from build123d import *

# Parameters (mm, degrees)
SKETCH1_R           = 75
BOSS_EXTRUDE1_DEPTH = 100
SHELL1_T            = -5
SKETCH3_R           = 20
SKETCH2_R           = 30
FILLET2_R           = 10


# Read off the part's stored shape, not the designer's step: Shell2
with BuildPart() as part:
    # Sketch1 → Boss-Extrude1 (new body)
    with BuildSketch(Plane(origin=(0, 0, 0), x_dir=(1, 0, 0), z_dir=(0, 1, 0))):
        with Locations(Location((0, 0, 0), (0, 0, 270))):
            Circle(SKETCH1_R)
    extrude(amount=BOSS_EXTRUDE1_DEPTH)

    # Shell1
    shell1_openings = [part.faces().sort_by_distance(p)[0] for p in [
        (0, 100, 0),
    ]]
    offset(amount=SHELL1_T, openings=shell1_openings, kind=Kind.INTERSECTION)

    # Sketch3 → Loft1 section 0
    with BuildSketch(Plane(origin=(0, 100, 0), x_dir=(1, 0, 0), z_dir=(0, 1, 0))):
        Circle(SKETCH3_R)
    # Sketch2 → Loft1 section 1
    with BuildSketch(Plane.XZ):
        Circle(SKETCH2_R)
    loft()

    # Shell2 outline → Shell2 (revolve, cut)
    with BuildSketch(Plane.XY):
        Polygon((0, 0), (24.975062189, 0), (14.975062189, 100), (0, 100), align=None)
    revolve(axis=Axis((0, 0, 0), (0, 1, 0)), mode=Mode.SUBTRACT)

    # Fillet1
    # an asymmetric fillet: 30, 5 mm, written as the material it takes off along each edge
    with BuildSketch(Plane(origin=(0, 0, 0), x_dir=(1, 0, 0), z_dir=(0, 0, 1))) as fillet1_piece_1:
        with BuildLine():
            Bezier((54.624689052, 0), (24.975062189, 0), (24.773573346, 2.014888429), weights=[1, 0.741452534, 1])
            Line((24.773573346, 2.014888429), (24.975062189, 0))
            Line((24.975062189, 0), (54.624689052, 0))
        make_face()
    revolve(axis=Axis((0, 0, 0), (0, 1, 0)), mode=Mode.SUBTRACT)

    # Fillet2
    fillet2_edges = [part.edges().sort_by_distance(p)[0] for p in [
        (-29.5, 5, 0),
    ]]
    fillet(fillet2_edges, radius=FILLET2_R)


solid = part.part
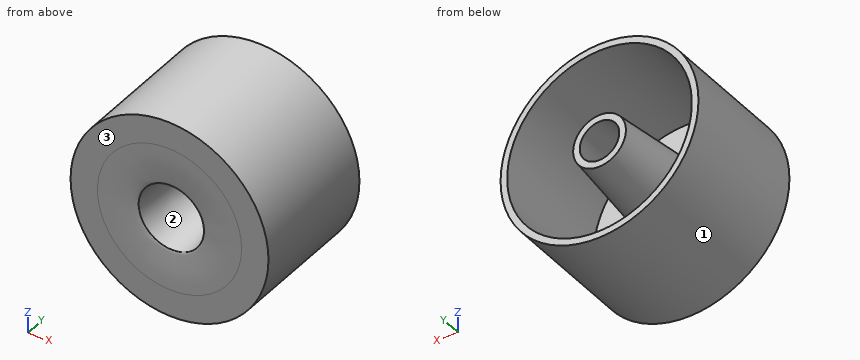
Work out the finished part from the listing and answer in its coordinate system (mm). Face numbers are marked on the shaded views. Coordinates: 2 decimals unless noted, no trailing zeros. Loops run counter-clockwise (first coordinate to the right, second up) from the corner with the lowest first, then second, coordinate; pieces in that order, holes last. Notation, with made-up numbers: (49, 34.5) -> (67, 34.5) arc R24 cw to (67, 44.5) -> close; hole circle Ø11 at (81, 11.25). An arc over 180 degrees is marked (long way). Write each question's results on one line, items separated by ' | '. Start each with the question number.
1) The mould has two halves that part along Z. Classify the marked faces 1, 2 and 3: pulls with the +Z half, pulls with the -Z half, needs draft (parallel to the pull), parting line crosses it, or undercut.
2) Find section B-B on x = -57. Determine the outline of the cut face in (y, z).
3) Flat-ended cylindrical pins translate along their axes: P1, Ø6, axis at x = -32.5, y = 52.5, coming from the -Z side; P2, Ø5, axis at y = 33.5, z = -24.5, coming from the -X side; P3, Ø8, axis at x = 29, z = 45.5, coming from the +Y side; P4, Ø2, axis at x = 36, z = -59, coming from the +Y side. Find the tip coordinate at first contact, or state that the pin passes through.
4) Consider line 1 along X through (y, z) = (92, -5.5); line 2 along X through (y, z) = (67, 0); line 3 along Z through (x, y) = (25.5, 15). Determine where each line is inside the solid, lowest interval first.
5) Find section A-A on y = 69. Determine the outline of the cut face in (x, z), then the cut area to 3 significant figures.
Response values:
1) face 1: parting line crosses it | face 2: undercut | face 3: needs draft
2) outline: (0, -48.74) -> (100, -48.74) -> (100, -40.63) -> (5, -40.63) -> (5, 40.63) -> (100, 40.63) -> (100, 48.74) -> (0, 48.74) -> close
3) P1: stops at z = -68.95 | P2: stops at x = -71.7 | P3: stops at y = 5 | P4: stops at y = 100
4) line 1: x = -74.8 to -69.78, -20.06 to -14.79, 14.79 to 20.06, 69.78 to 74.8 | line 2: x = -75 to -70, -23.3 to -18.28, 18.28 to 23.3, 70 to 75 | line 3: z = -70.53 to -65.19, -12.73 to 12.73, 65.19 to 70.53
5) outline: circle Ø150 at (0, 0); circle Ø46.2 at (0, 0); hole circle Ø140 at (0, 0); hole circle Ø36.15 at (0, 0) | area: 2,930 mm^2
